```python
from build123d import *

# Parameters (mm, degrees)
SKETCH1_W                                         = 63.5
SKETCH1_H                                         = 152.4
BOSS_EXTRUDE1_DEPTH                               = 3.175
F_6_CLEARANCE_HOLE1_D                             = 4.3053
F_6_CLEARANCE_HOLE1_DEPTH                         = 3.175
F_6_CLEARANCE_HOLE2_D                             = 4.3053
F_6_CLEARANCE_HOLE2_DEPTH                         = 3.175
F_1_2_0_5_DIAMETER_HOLE1_D                        = 12.7
F_1_2_0_5_DIAMETER_HOLE1_DEPTH                    = 3.175
F_9_64_0_14063_DIAMETER_HOLE1_D                   = 3.572002
F_9_64_0_14063_DIAMETER_HOLE1_DEPTH               = 3.175
F_19_64_0_29688_DIAMETER_HOLE1_D                  = 7.540752
F_19_64_0_29688_DIAMETER_HOLE1_DEPTH              = 3.175
CSK_FOR_6_FLAT_HEAD_MACHINE_SCREW_100_D           = 4.3053
CSK_FOR_6_FLAT_HEAD_MACHINE_SCREW_100_DEPTH       = 3.175
CSK_FOR_6_FLAT_HEAD_MACHINE_SCREW_100_CSINK_D     = 7.0866
CSK_FOR_6_FLAT_HEAD_MACHINE_SCREW_100_CSINK_ANGLE = 100
F_3_32_0_09375_DIAMETER_HOLE1_D                   = 2.38125
F_3_32_0_09375_DIAMETER_HOLE1_DEPTH               = 3.175


with BuildPart() as part:
    # Sketch1 → Boss-Extrude1 (new body)
    with BuildSketch(Plane.XY):
        with Locations((0, -76.2)):
            Rectangle(SKETCH1_W, SKETCH1_H)
    extrude(amount=-BOSS_EXTRUDE1_DEPTH)

    # #6 Clearance Hole1
    with Locations(Plane.XY):
        with Locations((-26.8605, -14.2875), (26.8605, -14.2875), (26.8605, -128.5875), (-26.8605, -128.5875)):
            Hole(F_6_CLEARANCE_HOLE1_D / 2, depth=F_6_CLEARANCE_HOLE1_DEPTH)

    # #6 Clearance Hole2
    with Locations(Plane.XY):
        with Locations((-23.495, -96.8375), (23.495, -96.8375), (-14.605, -13.208)):
            Hole(F_6_CLEARANCE_HOLE2_D / 2, depth=F_6_CLEARANCE_HOLE2_DEPTH)

    # 1/2 (0.5) Diameter Hole1
    with Locations(Plane.XY):
        with Locations((11.684, -79.375), (0, -120.65)):
            Hole(F_1_2_0_5_DIAMETER_HOLE1_D / 2, depth=F_1_2_0_5_DIAMETER_HOLE1_DEPTH)

    # 9/64 (0.14063) Diameter Hole1
    with Locations(Plane.XY):
        with Locations((0, -111.125), (11.684, -69.85)):
            Hole(F_9_64_0_14063_DIAMETER_HOLE1_D / 2, depth=F_9_64_0_14063_DIAMETER_HOLE1_DEPTH)

    # 19/64 (0.29688) Diameter Hole1
    with Locations(Plane.XY):
        with Locations((-15.24, -60.325), (6.35, -20.32)):
            Hole(F_19_64_0_29688_DIAMETER_HOLE1_D / 2, depth=F_19_64_0_29688_DIAMETER_HOLE1_DEPTH)

    # CSK for #6 Flat Head Machine Screw (100)1
    with Locations(Plane.XY):
        with Locations((-21.99, -72.39), (-21.99, -27.94), (22.46, -27.94)):
            CounterSinkHole(CSK_FOR_6_FLAT_HEAD_MACHINE_SCREW_100_D / 2, CSK_FOR_6_FLAT_HEAD_MACHINE_SCREW_100_CSINK_D / 2, depth=CSK_FOR_6_FLAT_HEAD_MACHINE_SCREW_100_DEPTH, counter_sink_angle=CSK_FOR_6_FLAT_HEAD_MACHINE_SCREW_100_CSINK_ANGLE)

    # 3/32 (0.09375) Diameter Hole1
    with Locations(Plane.XY):
        with Locations((-15.688380535, -54.341777215), (5.901619465, -14.336777215)):
            Hole(F_3_32_0_09375_DIAMETER_HOLE1_D / 2, depth=F_3_32_0_09375_DIAMETER_HOLE1_DEPTH)


solid = part.part
```
Check sheet for the modelled part. Datum: model origin and axes. Units: mm. Round coordinates to 2 decimals unless told otherwise and drop trailing zeros. Order: outer loops, then holes, each group sorted by start corner. A loop starts at its lowest first (then second) coordinate and runs counter-clockwise, first axis right, second up. Notation, with made-up numbers: (-37, 58.25) -> (-27, 58.25) arc R28 cw to (-27, 89.25) -> close; hole circle Ø4 at (14.25, 7.5). An arc over 180 degrees is marked (long way). One line per item, written item: value. Start each with the question number.
Q1. Cross-section at B-B (x = 15). Record the boundary of the cut face in (y, z) (3 decimals).
Q2. Cross-section at A-A (y = -20.32). Record the boundary of the cut face in (x, z) (3 decimals).
Q3. Thickness scan on line 1 (Y direction, x = -14, z = -1.95); line 2 (Y direction, x = -21, z = -0.9); line 3 (Y direction, x = -21.99, z = -1.7). Record the ranges inside material, lowest first.
Q4. Cross-section at C-C (z = -0.65). Give the number of separate pieces and of enclosed holes in the cut face, and give its area (3 significant figures).
Q5. Mould release check, pull along X, two halves, no side actions. Record for faces 1 (the face through (31.75, -77, -2)), 2 (the face through (0, -75, 0)), 3 (the face through (-18.836, -59.192, -1.61)): pulls with the +X half, pulls with the -X half, needs draft (parallel to the pull), parting line crosses it, or undercut.
Completed:
1. outline: (-152.4, -3.175) -> (-84.79, -3.175) -> (-84.79, 0) -> (-152.4, 0) -> close; (-73.96, -3.175) -> (0, -3.175) -> (0, 0) -> (-73.96, 0) -> close
2. outline: (-31.75, -3.175) -> (2.58, -3.175) -> (2.58, 0) -> (-31.75, 0) -> close; (10.12, -3.175) -> (31.75, -3.175) -> (31.75, 0) -> (10.12, 0) -> close
3. line 1: y = -152.4 to -63.89, -56.76 to -15.27, -11.14 to 0
3. line 2: y = -152.4 to -74.65, -70.13 to -30.2, -25.68 to 0
3. line 3: y = -152.4 to -98.38, -95.3 to -74.54, -70.24 to -30.09, -25.79 to 0
4. separate pieces: 1
4. enclosed holes: 18
4. area: 9,130 mm²
5. face 1: pulls with the +X half
5. face 2: needs draft
5. face 3: undercut
